Design review of the part built by this model. Coordinates are the model's own, in mm. Face numbers are marked on the shaded views. A direction names the side the tool comes from. Round coordinates to 2 decimals unless told otherwise and drop trailing zeros. Order: outer loops, then holes, each group sorted by start corner. A loop starts at its lowest first (then second) coordinate and runs counter-clockwise, first axis right, second up.
from build123d import *

# Parameters (mm, degrees)
ESQUISSE1_R             = 12
BOSS_EXTRU_1_DEPTH      = 20.5
ESQUISSE2_R             = 2.5
BOSS_EXTRU_2_DEPTH      = 2
ESQUISSE3_R             = 1.6
ENL_V_MAT_EXTRU_1_DEPTH = 3
ESQUISSE4_R             = 2.5
BOSS_EXTRU_3_DEPTH      = 8


with BuildPart() as part:
    # Esquisse1 → Boss.-Extru.1 (new body)
    with BuildSketch(Plane.XY):
        Circle(ESQUISSE1_R)
    extrude(amount=BOSS_EXTRU_1_DEPTH)

    # Esquisse2 → Boss.-Extru.2 (add)
    with BuildSketch(Plane.XY.offset(20.5)):
        Circle(ESQUISSE2_R)
    extrude(amount=BOSS_EXTRU_2_DEPTH)

    # Esquisse3 → Enlèv. mat.-Extru.1 (cut)
    with BuildSketch(Plane.XY.offset(20.5)):
        with Locations((0, 9)):
            Circle(ESQUISSE3_R)
        with Locations((-7.794228634, -4.5)):
            Circle(ESQUISSE3_R)
        with Locations((7.794228634, -4.5)):
            Circle(ESQUISSE3_R)
    extrude(amount=-ENL_V_MAT_EXTRU_1_DEPTH, mode=Mode.SUBTRACT)

    # Esquisse4 → Boss.-Extru.3 (add)
    with BuildSketch(Plane.XY.offset(22.5)):
        Circle(ESQUISSE4_R)
    extrude(amount=BOSS_EXTRU_3_DEPTH)


solid = part.part
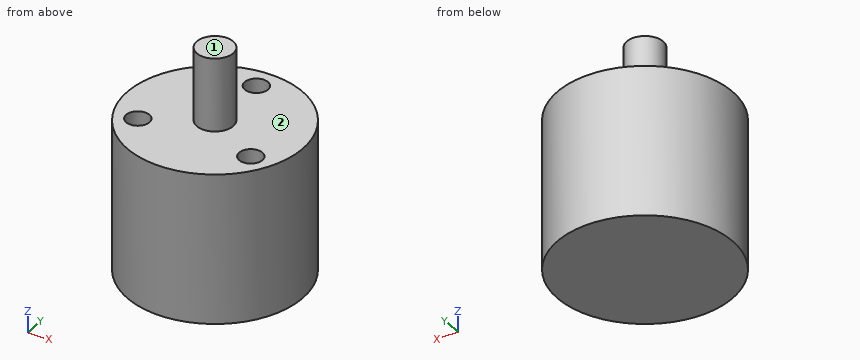
1) Take a section at C-C on z = 25.5. Give the boundary of the cut face in (x, y).
Results:
outline: circle Ø5 at (0, 0)
2) To check wall thickness, follow line 1 along Y through (x, z) = (0, 18.2); line 2 along Z through (x, y) = (-8.25, 8.25); line 3 along Z through (x, y) = (8.5, -3.5). State the ranges of each line that lie inside material, in increasing order.
Results:
line 1: y = -12 to 7.4, 10.6 to 12
line 2: z = 0 to 20.5
line 3: z = 0 to 17.5
3) Clearance check with flat-ended pins moving along their axes: P1, Ø6, axis at x = -6, z = 4.5, coming from the +Y side; P2, Ø3.5, axis at x = 7.79, y = -4.5, coming from the +Z side; P3, Ø1, axis at x = 0.5, y = 9.5, coming from the +Z side. State where each tip first meets the part, or that it passes through.
Results:
P1: stops at y = 11.62
P2: stops at z = 20.5
P3: stops at z = 17.5
4) Take a section at D-D on y = 9. Give the boundary of the cut face in (x, z), plus the area to 3 significant figures.
Results:
outline: (-7.94, 0) - (7.94, 0) - (7.94, 20.5) - (1.6, 20.5) - (1.6, 17.5) - (-1.6, 17.5) - (-1.6, 20.5) - (-7.94, 20.5) - close
area: 316 mm2
5) Take a section at A-A on x = 0. Give the boundary of the cut face in (y, z).
Results:
outline: (-12, 0) - (12, 0) - (12, 20.5) - (10.6, 20.5) - (10.6, 17.5) - (7.4, 17.5) - (7.4, 20.5) - (2.5, 20.5) - (2.5, 30.5) - (-2.5, 30.5) - (-2.5, 20.5) - (-12, 20.5) - close
6) Take a section at B-B on y = 0. Give the boundary of the cut face in (x, z), plus the area to 3 significant figures.
Results:
outline: (-12, 0) - (12, 0) - (12, 20.5) - (2.5, 20.5) - (2.5, 30.5) - (-2.5, 30.5) - (-2.5, 20.5) - (-12, 20.5) - close
area: 542 mm2
7) For the marked faces 1 and 2, list the 3-axis set-ups (+Z, -Z, +X, -X, +Y, -Y) from which the entire face can be reached by the end or side of a thin tool; tool diameter is ignored.
Results:
face 1: +Z, +X, -X, +Y, -Y
face 2: +Z
